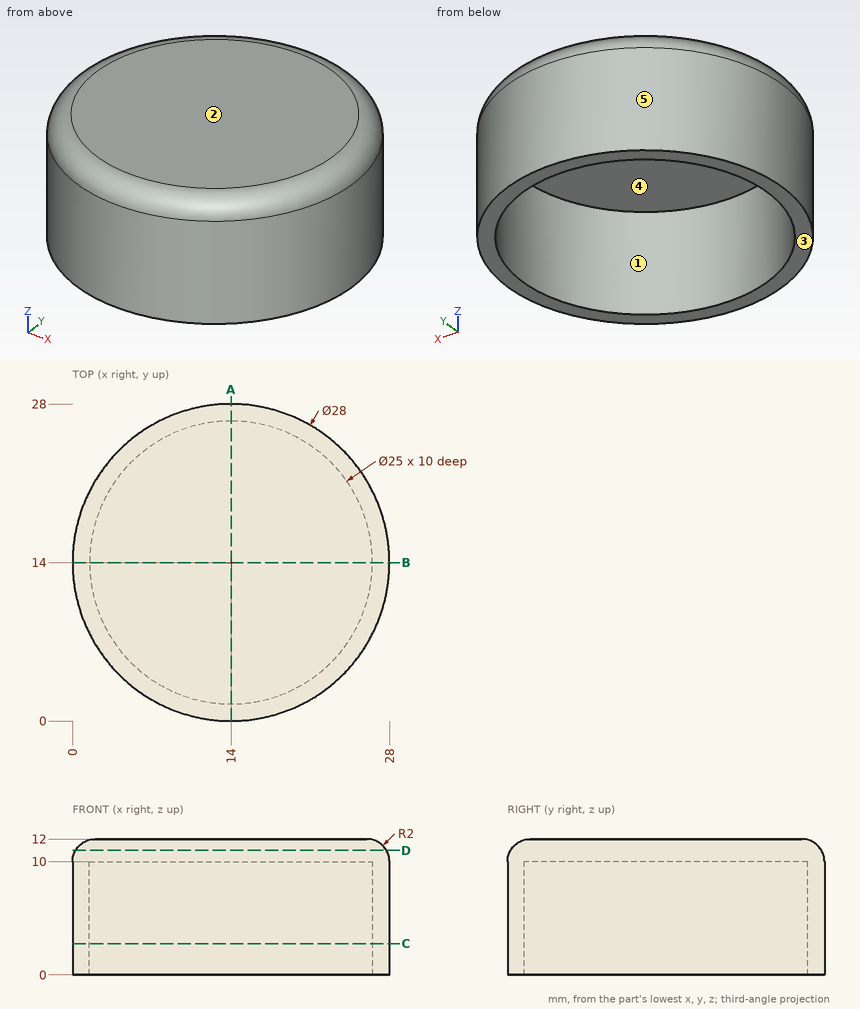
Input: dimensioned drawing with shaded views. Units: mm. Origin: part minimum x, y, z. A direction names the side the tool comes from. Round coordinates to 2 decimals unless told otherwise and drop trailing zeros. Loops run counter-clockwise (first coordinate to the right, second up) from the corner with the lowest first, then second, coordinate; pieces in that order, holes last. Notation, with made-up numbers: (-34.5, 87.5) -> (13.5, 87.5) arc R25 cw to (13.5, 103.5) -> close; hole circle Ø4 at (2.25, 40). An arc over 180 degrees is marked (long way). Use one line per item in the form item = value. Start each with the question number.
1) Section C-C on z = 2.75. Output: boundary loops of the cut face in (x, y).
2) Draft query along Y for the marked faces 3, 4 and 5. Return one class per face: released by +Y, released by -Y, zero draft, split by the parting line, or undercut.
3) Section A-A on x = 14. Output: boundary loops of the cut face in (y, z).
4) Access query for the marked faces 1 and 2. Directions: +Z, -Z, +X, -X, +Y, -Y. A direction counts if a zero-diameter tool reaches every point of the face in a straight line with its end or side. Return the directions, or none.
5) First-contact query: P1, Ø5, axis at y = 4.5, z = 5, coming from the -X side; P2, Ø4, axis at y = 21, z = 4.5, coming from the -X side; P3, Ø1.5, axis at y = 22.5, z = 10, coming from the +X side. Flat tips, straight axial feed; report the tip coordinate or a pass-through.
6) Line query: L1, parallel to Y at x = 14, z = 6.5; L2, parallel to Z at x = 5.75, y = 9.5; L3, parallel to Y at x = 6.75, z = 2.75. Output: solid intervals per line, ascending.
7) Section D-D on z = 11. Output: boundary loops of the cut face in (x, y), then the cut area to 3 significant figures.
Response:
q1.outline = circle Ø28 at (14, 14); hole circle Ø25 at (14, 14)
q2.face_3 = zero draft
q2.face_4 = undercut
q2.face_5 = split by the parting line
q3.outline = (0, 0) -> (1.5, 0) -> (1.5, 10) -> (26.5, 10) -> (26.5, 0) -> (28, 0) -> (28, 10) arc R2 ccw to (26, 12) -> (2, 12) arc R2 ccw to (0, 10) -> close
q4.face_1 = -Z
q4.face_2 = +Z, +X, -X, +Y, -Y
q5.P1 = 1.88
q5.P2 = 0.92
q5.P3 = 25.66
q6.L1 = 0 to 1.5, 26.5 to 28
q6.L2 = 10 to 12
q6.L3 = 2.02 to 3.82, 24.18 to 25.98
q7.outline = circle Ø27.46 at (14, 14)
q7.area = 592 mm^2
